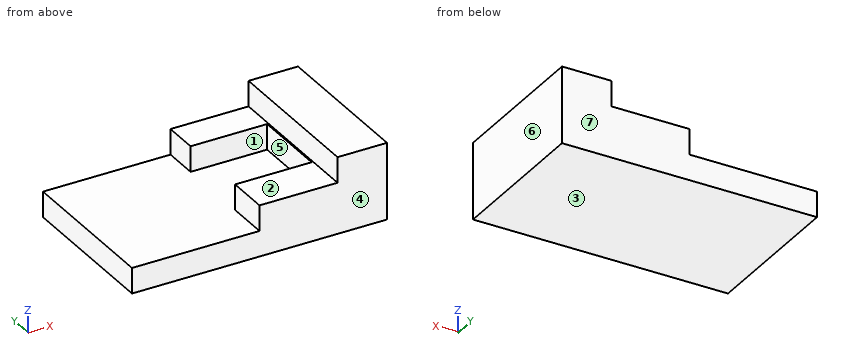
```python
from build123d import *

# Parameters (mm, degrees)
F0_W     = 127
F0_H     = 76.2
F1_DEPTH = 12.7
F2_W     = 63.5
F2_H     = 76.2
F3_DEPTH = 12.7
F4_W     = 38.1
F4_H     = 38.1
F5_DEPTH = 12.7
F6_W     = 24.64416
F6_H     = 76.2
F7_DEPTH = 12.7


with BuildPart() as f1:
    # F0 (on Top) → F1 (new body)
    with BuildSketch(Plane.XY):
        Rectangle(F0_W, F0_H)
    extrude(amount=F1_DEPTH)

    # F2 (on face) → F3 (join)
    with BuildSketch(Plane.XY.offset(12.7)):
        with Locations((31.75, 0)):
            Rectangle(F2_W, F2_H)
    extrude(amount=F3_DEPTH)

    # F4 (on face) → F5 (cut)
    with BuildSketch(Plane.XY.offset(25.4)):
        with Locations((19.05, 1.858458)):
            Rectangle(F4_W, F4_H)
    extrude(amount=-F5_DEPTH, mode=Mode.SUBTRACT)

    # F6 (on face) → F7 (join)
    with BuildSketch(Plane.XY.offset(25.4)):
        with Locations((51.17792, 0)):
            Rectangle(F6_W, F6_H)
    extrude(amount=F7_DEPTH)


solid = f1.part
```
Work out the finished part from the listing and answer in its coordinate system (mm). Face numbers are marked on the shaded views. A direction names the side the tool comes from. Give positions to 0.01 mm unless a question says otherwise; leave off trailing zeros. Order: outer loops, then holes, each group sorted by start corner. A loop starts at its lowest first (then second) coordinate and runs counter-clockwise, first axis right, second up. Notation, with made-up numbers: (41, 71.5) - (58, 71.5) arc R16 cw to (58, 94.5) - close; hole circle Ø10 at (-37, 75.5). An arc over 180 degrees is marked (long way). One line per item, written item: value. Start each with the question number.
1. Consider line 1 (X direction, y = -34, z = 28); line 2 (Y direction, x = 27, z = 13); line 3 (Z direction, x = -42.5, y = 1). Determine where each line is inside the solid, lowest interval first.
2. Which of the six approach directions +Z, -Z, +X, -X, +Y, -Y give full straight-line access (tool end or side, diameter ignored) to the marked faces 1, 2 and 3?
3. Section D-D, the plane x = -41 is taken. Write down the section's boundary in (y, z), then the cut area to 3 significant figures.
4. Each of these flat-tipped pins is pushed along its axis until it touches: pin 1 Ø6.5 at (y, z) = (31.5, 17) entering from -X; pin 2 Ø6.5 at (y, z) = (-14, 29) entering from -X; pin 3 Ø3 at (x, y) = (-1.5, -12) entering from +Z. Where does it stop, or does it pass through?
5. Section A-A, the plane y = -19 is taken. Write down the section's boundary in (x, z).
6. Section C-C, the plane z = 27 is taken. Write down the section's boundary in (x, y).
7. Section B-B, the plane x = 12 is taken. Write down the section's boundary in (y, z), then the cut area to 3 significant figures.
8. For a pull along Y with two mould halves and no side action, classify the marked faces 4, 5, 6 and 7 as released by +Y, released by -Y, zero draft, split by the parting line, or undercut.
Filled sheet:
1. line 1: 38.86 to 63.5
1. line 2: -38.1 to -17.19, 20.91 to 38.1
1. line 3: 0 to 12.7
2. face 1: +Z, -X
2. face 2: +Z, -X, +Y, -Y
2. face 3: -Z, +X, -X, +Y, -Y
3. outline: (-38.1, 0) - (38.1, 0) - (38.1, 12.7) - (-38.1, 12.7) - close
3. area: 968 mm²
4. pin 1: x = 0
4. pin 2: x = 38.86
4. pin 3: z = 12.7
5. outline: (-63.5, 0) - (63.5, 0) - (63.5, 38.1) - (38.86, 38.1) - (38.86, 25.4) - (0, 25.4) - (0, 12.7) - (-63.5, 12.7) - close
6. outline: (38.86, -38.1) - (63.5, -38.1) - (63.5, 38.1) - (38.86, 38.1) - close
7. outline: (-38.1, 0) - (38.1, 0) - (38.1, 25.4) - (20.91, 25.4) - (20.91, 12.7) - (-17.19, 12.7) - (-17.19, 25.4) - (-38.1, 25.4) - close
7. area: 1,450 mm²
8. face 4: released by -Y
8. face 5: undercut
8. face 6: zero draft
8. face 7: released by +Y
